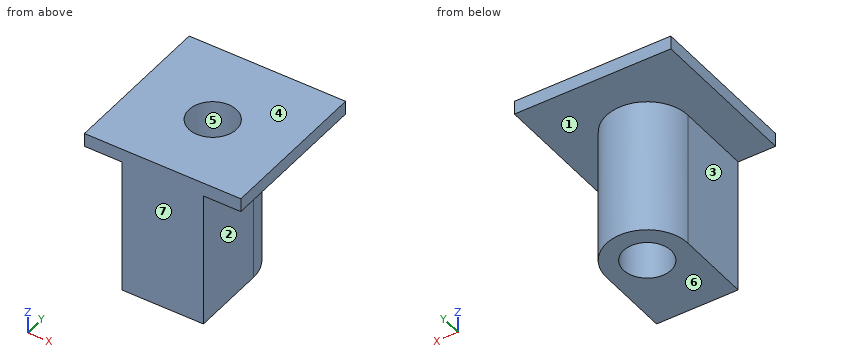
```python
from build123d import *

# Parameters (mm, degrees)
SKETCH022_W     = 11.5
SKETCH022_H     = 11.5
PAD010_DEPTH    = 1
PAD011_DEPTH    = 10
SKETCH024_R     = 1.75
POCKET010_DEPTH = 11.001


with BuildPart() as part:
    # Sketch022 → Pad010 (new body)
    with BuildSketch(Plane.XY):
        with Locations((0, 5.75)):
            Rectangle(SKETCH022_W, SKETCH022_H)
    extrude(amount=PAD010_DEPTH)

    # Sketch023 (on Face5 of Pad010) → Pad011 (join)
    with BuildSketch(Plane(origin=(0, 0, 0), x_dir=(1, 0, 0), z_dir=(0, 0, -1))):
        with BuildLine():
            Line((-3, -5.5), (-3, 0))
            Line((-3, 0), (3, 0))
            Line((3, 0), (3, -5.5))
            ThreePointArc((-3, -5.5), (0, -8.5), (3, -5.5))
        make_face()
    extrude(amount=PAD011_DEPTH)

    # Sketch024 (on Face11 of Pad011) → Pocket010 (cut, through all)
    with BuildSketch(Plane(origin=(0, 0, -10), x_dir=(1, 0, 0), z_dir=(0, 0, -1))):
        with Locations((0, -5.5)):
            Circle(SKETCH024_R)
    extrude(amount=-POCKET010_DEPTH, mode=Mode.SUBTRACT)


with BuildPart() as part_1:
    # Body009 placement: moved
    add(part.part.moved(Location((0, 72.5, 28.2))))


solid = part_1.part
```
Input: part model. Units: mm. Frame: model coordinates. Face numbers are marked on the shaded views. A direction names the side the tool comes from. Round coordinates to 2 decimals unless told otherwise and drop trailing zeros. Loops run counter-clockwise (first coordinate to the right, second up) from the corner with the lowest first, then second, coordinate; pieces in that order, holes last. Notation, with made-up numbers: M 18.5,54.25 L 24.5,54.25 A27 ccw 24.5,87.25 Z; hole C -18.75,89 d6. An arc over 180 degrees is marked long. Answer in a Markdown table with one row per item. Add a question column.
1. Section D-D (x = -4.5). Output: boundary loops of the cut face in (y, z), and give its area (3 significant figures).
2. Section C-C (y = 76). Output: boundary loops of the cut face in (x, z).
3. Mould query, pull axis Y, two halves, no side actions, for the marked faces 5, 6 and 7. Classes: released by +Y, released by -Y, zero draft, split by the parting line, or undercut.
4. Contact query for flat-ended pins moving along their axis: pin 1 (4 mm diameter, centred on x = -0.5, z = 20.5, fed in from +Y); pin 2 (5.5 mm diameter, centred on x = 0, y = 78, fed in from -Z); pin 3 (1 mm diameter, centred on x = -2, z = 22.5, fed in from +Y); pin 4 (3 mm diameter, centred on y = 76, z = 23, fed in from -X). Output: stop coordinate, or through.
5. Ray query, probe 1 along X at (y, z) = (78, 24); probe 2 along Y at (x, z) = (0, 26.75); probe 3 along Z at (x, y) = (-4.5, 73.75). Return the intervals inside material, ascending.
6. Section B-B (z = 27). Output: boundary loops of the cut face in (x, y), and give its area (3 significant figures).
7. Set-up query: the marked faces 1, 2, 3 and 4. Return all of +Z, -Z, +X, -X, +Y, -Y with unobstructed straight access to the full face (end or side cutting, diameter ignored); none if empty.
8. Section A-A (x = 0). Output: boundary loops of the cut face in (y, z).
Values follow:
| question | item | result |
|---|---|---|
| 1 | outline | M 72.5,28.2 L 84,28.2 L 84,29.2 L 72.5,29.2 Z |
| 1 | area | 11.5 mm^2 |
| 2 | outline | M -5.75,28.2 L -3,28.2 L -3,18.2 L 3,18.2 L 3,28.2 L 5.75,28.2 L 5.75,29.2 L -5.75,29.2 Z |
| 3 | face 5 | undercut |
| 3 | face 6 | zero draft |
| 3 | face 7 | released by -Y |
| 4 | pin 1 | y = 81 |
| 4 | pin 2 | z = 18.2 |
| 4 | pin 3 | y = 80.6 |
| 4 | pin 4 | x = -3 |
| 5 | probe 1 | -3 to -1.75, 1.75 to 3 |
| 5 | probe 2 | 72.5 to 76.25, 79.75 to 81 |
| 5 | probe 3 | 28.2 to 29.2 |
| 6 | outline | M -3,72.5 L 3,72.5 L 3,78 A3 ccw -3,78 Z; hole C 0,78 d3.5 |
| 6 | area | 37.5 mm^2 |
| 7 | face 1 | -Z, +Y |
| 7 | face 2 | -Z, +X, +Y, -Y |
| 7 | face 3 | -Z, -X, +Y, -Y |
| 7 | face 4 | +Z, +X, -X, +Y, -Y |
| 8 | outline | M 72.5,18.2 L 76.25,18.2 L 76.25,29.2 L 72.5,29.2 Z; M 79.75,18.2 L 81,18.2 L 81,28.2 L 84,28.2 L 84,29.2 L 79.75,29.2 Z |
